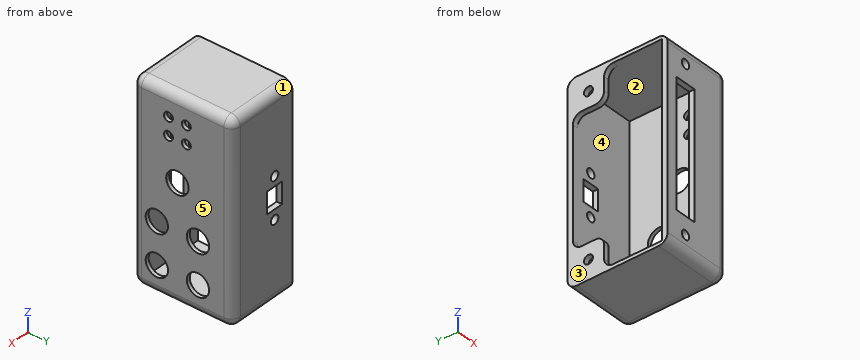
Autodesk Inventor part; units mm, degrees
ref_plane "YZ Plane" through (0, 0, 0) normal (1, 0, 0) x (0, 1, 0)
ref_plane "XZ Plane" through (0, 0, 0) normal (0, 1, 0) x (-1, 0, 0)
ref_plane "XY Plane" through (0, 0, 0) normal (0, 0, 1) x (1, 0, 0)
sketch "Sketch1" plane through (0, 0, 0) normal (0, 1, 0) x (-1, 0, 0)
  circle A0 centre (0, 45) radius 2.5
  circle A1 centre (0, -45) radius 2.5
  line L0 (12, 55) -> (-28, 55)
  line L1 (-28, 55) -> (-28, -55)
  line L2 (-28, -55) -> (12, -55)
  line L3 (12, -55) -> (12, 55)
  line L4 (-6, -35) -> (6, -35)
  line L5 (6, -35) -> (6, 35)
  line L6 (6, 35) -> (-6, 35)
  line L7 (-6, 35) -> (-6, -35)
  point P0 (0, 0)
  point P1 (0, -35)
  point P2 (0, 35)
  dimension "d0" = 5
  dimension "d1" = 5
  dimension "d2" = 90
  dimension "d3" = 45
  dimension "d4" = 40
  dimension "d6" = 110
  dimension "d7" = 55
  dimension "d36" = 70
  dimension "d37" = 12
  dimension "d38" = 35
  dimension "d39" = 0
  dimension "d40" = 28
  dimension "d42" = 0
  dimension "d52" = 0
extrude "Extrusion1" add sketch "Sketch1" along normal blind 3
sketch "Sketch2" plane through (0, 3, 0) normal (0, 1, 0) x (1, 0, 0)
  line L0 (-12, -55) -> (28, -55)
  line L1 (-12, 55) -> (-12, -55)
  line L2 (28, -55) -> (-12, -55)
  line L3 (-12, -55) -> (-12, -53)
  line L4 (-12, -53) -> (28, -53)
  line L5 (28, -53) -> (28, -55)
  line L6 (28, 55) -> (-12, 55)
  line L7 (28, -55) -> (26, -55)
  line L8 (26, -55) -> (26, 55)
  line L9 (26, 55) -> (28, 55)
  line L10 (28, 55) -> (28, -55)
  line L11 (28, 55) -> (-12, 55)
  line L12 (-12, 55) -> (-12, 53)
  line L13 (-12, 53) -> (28, 53)
  line L14 (28, 53) -> (28, 55)
  point P0 (0, 0)
  point P1 (-12, 53)
  point P2 (26, 53)
  point P3 (26, -53)
  dimension "d10" = 2
  dimension "d11" = 2
  dimension "d12" = 2
extrude "Extrusion2" add sketch "Sketch2" along normal blind 50 contours L1 L4 L8 L0 | L8 L4 L5 L0 | L8 L13 L10 L4 | L1 L6 L8 L13 | L8 L6 L10 L13
sketch "Sketch3" plane through (28, 0, 55) normal (1, 0, 0) x (0, 0, -1)
  line L0 (94.5, 13.5) -> (71.5, 13.5)
  line L1 (71.5, 13.5) -> (71.5, 36.5)
  line L2 (71.5, 36.5) -> (94.5, 36.5)
  line L3 (94.5, 36.5) -> (94.5, 13.5)
  line L4 (94.5, 13.5) -> (71.5, 36.5) construction
  line L5 (71.5, 13.5) -> (94.5, 36.5) construction
  circle A0 centre (94.5, 13.5) radius 6.25
  circle A1 centre (71.5, 13.5) radius 6.25
  circle A2 centre (94.5, 36.5) radius 6.25
  circle A3 centre (71.5, 36.5) radius 6.25
  line L6 (23.5, 20) -> (13.5, 20)
  line L7 (13.5, 20) -> (13.5, 30)
  line L8 (13.5, 30) -> (23.5, 30)
  line L9 (23.5, 30) -> (23.5, 20)
  line L10 (23.5, 20) -> (13.5, 30) construction
  line L11 (13.5, 20) -> (23.5, 30) construction
  circle A4 centre (23.5, 20) radius 2.5
  circle A5 centre (13.5, 20) radius 2.5
  circle A6 centre (13.5, 30) radius 2.5
  circle A7 centre (23.5, 30) radius 2.5
  circle A8 centre (46, 25) radius 6.25
  line L12 (0, 0) -> (110, 0)
  line L13 (110, 0) -> (110, 53)
  point P0 (55, 0)
  point P1 (83, 25)
  point P2 (18.5, 25)
  dimension "d15" = 23
  dimension "d16" = 23
  dimension "d17" = 12.5
  dimension "d18" = 12.5
  dimension "d19" = 12.5
  dimension "d20" = 12.5
  dimension "d21" = 10
  dimension "d22" = 10
  dimension "d23" = 5
  dimension "d24" = 5
  dimension "d25" = 5
  dimension "d26" = 5
  dimension "d27" = 12.5
  dimension "d28" = 25
  dimension "d29" = 25
  dimension "d30" = 25
  dimension "d31" = 27
  dimension "d32" = 37
  dimension "d33" = 27.5
extrude "Extrusion3" cut sketch "Sketch3" against normal through all contours A1 L1 L0 | L0 L1 A1 | A0 L3 L0 | L0 L3 A0 | A3 L2 L1 | L1 L2 A3 | A2 L2 L3 | L3 L2 A2 | A5 L7 L6 | L6 L7 A5 | A4 L9 L6 | L6 L9 A4 | A6 L8 L7 | L7 L8 A6 | A7 L8 L9 | L9 L8 A7 | A8
sketch "Sketch4" plane through (0, 53, 0) normal (0, 1, 0) x (1, 0, 0)
  line L0 (28, 55) -> (-12, 55)
  line L1 (28, 55) -> (-12, 55)
  line L2 (-12, 55) -> (-12, -55)
  line L3 (-12, -55) -> (28, -55)
  line L4 (28, -55) -> (28, 55)
  line L5 (5, 6) -> (-5, 6)
  line L6 (-5, 6) -> (-5, -6)
  line L7 (-5, -6) -> (5, -6)
  line L8 (5, -6) -> (5, 6)
  line L9 (5, 6) -> (-5, -6) construction
  line L10 (-5, 6) -> (5, -6) construction
  circle A0 centre (0, 11.5) radius 2.5
  circle A1 centre (0, -11.5) radius 2.5
  point P0 (0, 0)
  dimension "d43" = 10
  dimension "d44" = 12
  dimension "d45" = 5
  dimension "d46" = 5
  dimension "d47" = 23
  dimension "d48" = 11.5
extrude "Extrusion4" add sketch "Sketch4" along normal blind 3
fillet "Fillet1" radius 5 8 edges at (28, 0, 0) (28, 28, -55) (8, 0, -55) (8, 0, 55) (28, 28, 55) (28, 56, 0) (8, 56, -55) (8, 56, 55)
sketch "Sketch5" plane through (-12, 0, -50) normal (-1, 0, 0) x (0, 0, 1)
  line L0 (-3, 53) -> (103, 53)
  line L1 (103, 53) -> (85.5, 53)
  line L2 (85.5, 53) -> (85.5, 35.5)
  line L3 (85.5, 35.5) -> (103, 35.5)
  line L4 (103, 35.5) -> (103, 53)
  line L5 (-3, 53) -> (14.5, 53)
  line L6 (14.5, 53) -> (14.5, 35.5)
  line L7 (14.5, 35.5) -> (-3, 35.5)
  line L8 (-3, 35.5) -> (-3, 53)
  circle A0 centre (94.25, 44.25) radius 2.5
  circle A1 centre (5.75, 44.25) radius 2.5
  point P0 (50, 0)
  point P1 (14.5, 53)
  dimension "d54" = 17.5
  dimension "d55" = 17.5
  dimension "d56" = 17.5
  dimension "d57" = 17.5
  dimension "d58" = 5
  dimension "d59" = 5
  dimension "d60" = 8.75
  dimension "d61" = 8.75
  dimension "d62" = 8.75
  dimension "d63" = 8.75
extrude "Extrusion5" add sketch "Sketch5" against normal blind 3
fillet "Fillet2" radius 5 6 edges at (-10.5, 35.5, 53) (-10.5, 35.5, 35.5) (-10.5, 53, 35.5) (-10.5, 53, -35.5) (-10.5, 35.5, -35.5) (-10.5, 35.5, -53)
properties part number "electro_hold"
Geometry: final body of the model. Coordinates: model frame, mm. Face numbers are marked on the shaded views. A direction names the side the tool comes from. Round coordinates to 2 decimals unless told otherwise and drop trailing zeros. Write each loop counter-clockwise with the first axis right and the second up, starting at its lowest first coordinate (ties: lowest second). Pieces come first, ordered by that corner, then holes.
Item 1: Section query D-D (x = 0). Give the number of separate pieces and of enclosed holes in the cut face, plus the area to 3 significant figures.
Item 2: Pin query (flat end, axial travel): P1, Ø11, axis at y = 13.5, z = -16.5, coming from the -X side; P2, Ø4.5, axis at y = 44.25, z = -44.25, coming from the -X side; P3, Ø0.9, axis at x = -1, y = 54.5, coming from the +Z side. Return the tip coordinate at first contact, or that it passes through.
Item 3: Section query C-C (z = 17.5). Return loops of the section in (x, y).
Item 4: Section query A-A (y = 44.25). Return loops of the section in (x, z), plus the area to 3 significant figures.
Item 5: Set-up query: the marked faces 4 and 5. Return all of +Z, -Z, +X, -X, +Y, -Y with unobstructed straight access to the full face (end or side cutting, diameter ignored); none if empty.
Item 6: Material intervals for L1, parallel to Z at x = -10, y = 44; L2, parallel to Z at x = -2.5, y = 49; L3, parallel to X at y = 45, z = 39.5, sorted ascending.
Item 7: Mould query, pull axis X, two halves, no side actions, for the marked faces 1, 2 and 3. Classes: +X half, -X half, draft (parallel to the pull), parting line (faces both ways), or undercut.
Item 8: Section query B-B (y = 25). Return loops of the section in (x, z).
Completed:
1. separate pieces: 6
1. enclosed holes: 0
1. area: 533 mm2
2. P1: passes through
2. P2: stops at x = 26
2. P3: stops at z = 53.96
3. outline: (-12, 0) - (-6, 0) - (-6, 3) - (-12, 3) - close; (-12, 53) - (26, 53) - (26, 3) - (6, 3) - (6, 0) - (23, 0) arc R5 ccw to (28, 5) - (28, 51) arc R5 ccw to (23, 56) - (-12, 56) - close
4. outline: (-12, -55) - (23, -55) arc R5 ccw to (28, -50) - (28, 50) arc R5 ccw to (23, 55) - (-12, 55) - (-12, 46.75) - (-9, 46.75) - (-9, 53) - (26, 53) - (26, -53) - (-9, -53) - (-9, -46.75) - (-12, -46.75) - close; (-12, -41.75) - (-9, -41.75) - (-9, -35.5) - (-12, -35.5) - close; (-12, 35.5) - (-9, 35.5) - (-9, 41.75) - (-12, 41.75) - close
4. area: 436 mm2
5. face 4: none
5. face 5: +Z, -Z, +X, +Y, -Y
6. L1: z = -55 to -46.74, -41.76 to -35.5, 35.5 to 41.76, 46.74 to 55
6. L2: z = -55 to -53, 53 to 55
6. L3: x = -12 to -9, 26 to 28
7. face 1: draft
7. face 2: undercut
7. face 3: -X half
8. outline: (-12, -55) - (23, -55) arc R5 ccw to (28, -50) - (28, 2.75) - (26, 2.75) - (26, -53) - (-12, -53) - close; (-12, 53) - (26, 53) - (26, 15.25) - (28, 15.25) - (28, 50) arc R5 ccw to (23, 55) - (-12, 55) - close
